Autodesk Inventor part; units mm, degrees
ref_plane "YZ Plane" through (0, 0, 0) normal (1, 0, 0) x (0, 1, 0)
ref_plane "XZ Plane" through (0, 0, 0) normal (0, 1, 0) x (-1, 0, 0)
ref_plane "XY Plane" through (0, 0, 0) normal (0, 0, 1) x (1, 0, 0)
sketch "Sketch1" plane through (0, 0, 0) normal (0, 1, 0) x (-1, 0, 0)
  point P0 (0, 0)
extrude "Extrusion1" [suppressed]
sketch "Sketch2" plane through (0, 0, 0) normal (1, 0, 0) x (0, 1, 0)
  arc A0 (-9.8478, -6.8571) -> (-9.8478, 6.8571) centre (0, 0) ccw
  line L0 (0, 0) -> (-30, 0)
  arc A1 (-30, 6) -> (-30, -6) centre (-30, 0) ccw
  line L1 (-30, -6) -> (-11.4891, -6)
  line L2 (-30, 6) -> (-11.4891, 6)
  arc A2 (-9.8478, -6.8571) -> (-11.4891, -6) centre (-11.4891, -8) ccw
  arc A3 (-11.4891, 6) -> (-9.8478, 6.8571) centre (-11.4891, 8) ccw
  line L3 (0, 0) -> (-28, 0)
  line L4 (-28, 0) -> (-28, -20)
  line L5 (-28, -20) -> (-28, 20)
  circle A4 centre (-28, -20) radius 5
  circle A5 centre (-28, 20) radius 5
  line L6 (0, 0) -> (22, 0)
  circle A6 centre (22, 0) radius 5
  circle A7 centre (22, 0) radius 10
  circle A8 centre (-28, -20) radius 10
  circle A9 centre (-28, 20) radius 10
  line L7 (25.7139, -9.2848) -> (-24.2861, -29.2848)
  line L8 (-38, -20) -> (-38, 20)
  line L9 (-24.2861, 29.2848) -> (25.7139, 9.2848)
  point P0 (-10.3923, -6)
  point P1 (-10.3923, 6)
  dimension "d15" = 24
  dimension "d16" = 30
  dimension "d17" = 12
  dimension "d18" = 2
  dimension "d19" = 28
  dimension "d20" = 20
  dimension "d21" = 40
  dimension "d22" = 10
  dimension "d23" = 10
  dimension "d24" = 22
  dimension "d25" = 10
  dimension "d26" = 20
  dimension "d27" = 20
  dimension "d28" = 20
extrude "Extrusion2" add sketch "Sketch2" along normal blind 10 contours A0 A7 L7 A8 L4 L1 A2 | A0 A3 L2 L5 A9 L9 A7 | A7 | L4 A8 L8 A9 L5 L2 A1 L1 | A9 | A8
equation "\"d10\" = 0.5 * d9"
Geometry: final body of the model. Coordinates: model frame, mm. A direction names the side the tool comes from. Round coordinates to 2 decimals unless told otherwise and drop trailing zeros. Order: outer loops, then holes, each group sorted by start corner. A loop starts at its lowest first (then second) coordinate and runs counter-clockwise, first axis right, second up.
Q1. Pin query (flat end, axial travel): pin 1 (14.5 mm diameter, centred on y = 0, z = 0, fed in from -X); pin 2 (2 mm diameter, centred on x = 8, y = 2.5, fed in from -Z); pin 3 (3 mm diameter, centred on x = 3, y = -16, fed in from +Z); pin 4 (3 mm diameter, centred on x = 5, y = -19, fed in from -Z). Return the tip coordinate at first contact, or that it passes through.
Result sheet:
pin 1: passes through
pin 2: stops at z = -18.97
pin 3: stops at z = 26.57
pin 4: stops at z = -27.77
Q2. Section D-D, the plane y = 11. Output: boundary loops of the cut face in (x, z), and give its area (3 significant figures).
Result sheet:
outline: (0, -15.17) - (10, -15.17) - (10, -4.8) - (0, -4.8) - close; (0, 4.8) - (10, 4.8) - (10, 15.17) - (0, 15.17) - close
area: 207 mm2
Q3. Material intervals for probe 1 along Z at (x, y) = (6.75, -28); probe 2 along Y at (x, z) = (7.25, 0); probe 3 along Y at (x, z) = (8.75, -4.5), sorted ascending.
Result sheet:
probe 1: z = -30 to -25, -15 to -6, 6 to 15, 25 to 30
probe 2: y = -38 to -36, 12 to 17, 27 to 32
probe 3: y = -38 to -33.97, 11.12 to 19.82, 24.18 to 30.93
Q4. Mould query, pull axis Z, two halves, no side actions, for faces 3 (the face through (5, -38, 0)), 4 (the face through (4.93, 0.364, 19.425)), 5 (the face through (5, -21, 6)), 6 (the face through (4.93, -33.49, -28.36)). Classes: released by +Z, released by -Z, zero draft, split by the parting line, or undercut.
Result sheet:
face 3: zero draft
face 4: released by +Z
face 5: undercut
face 6: released by -Z
Q5. Section C-C, the plane z = 23. Output: boundary loops of the cut face in (x, y), and give its area (3 significant figures).
Result sheet:
outline: (0, -37.54) - (10, -37.54) - (10, -32) - (0, -32) - close; (0, -24) - (10, -24) - (10, -8.57) - (0, -8.57) - close
area: 210 mm2
Q6. Section B-B, the plane z = 0. Output: boundary loops of the cut face in (x, y), and give its area (3 significant figures).
Result sheet:
outline: (0, -38) - (10, -38) - (10, -36) - (0, -36) - close; (0, 12) - (10, 12) - (10, 17) - (0, 17) - close; (0, 27) - (10, 27) - (10, 32) - (0, 32) - close
area: 120 mm2
Q7. Section A-A, the plane y = -28. Output: boundary loops of the cut face in (x, z).
Result sheet:
outline: (0, -30) - (10, -30) - (10, -25) - (0, -25) - close; (0, -15) - (10, -15) - (10, -6) - (0, -6) - close; (0, 6) - (10, 6) - (10, 15) - (0, 15) - close; (0, 25) - (10, 25) - (10, 30) - (0, 30) - close
Q8. Access query for faces 1 (the face through (5, -34, 28)), 2 (the face through (5, -21, -6)). Directions: +Z, -Z, +X, -X, +Y, -Y. A direction counts if a zero-diameter tool reaches every point of the face in a straight line with its end or side. Return the directions, or none.
Result sheet:
face 1: +Z, +X, -X
face 2: +X, -X
